Autodesk Inventor part; units mm, degrees
ref_plane "YZ Plane" through (0, 0, 0) normal (1, 0, 0) x (0, 1, 0)
ref_plane "XZ Plane" through (0, 0, 0) normal (0, 1, 0) x (-1, 0, 0)
ref_plane "XY Plane" through (0, 0, 0) normal (0, 0, 1) x (1, 0, 0)
sketch "Sketch1" plane through (0, 0, 0) normal (0, 0, 1) x (1, 0, 0)
  line L0 (0, 0) -> (35, 0)
  line L1 (35, 0) -> (35, 35)
  line L2 (35, 35) -> (0, 35)
  line L3 (0, 35) -> (0, 0)
  line L4 (17.5, 35) -> (17.5, 0)
  line L5 (0, 17.5) -> (35, 17.5)
  dimension "d0" = 35
  dimension "d1" = 35
extrude "Extrusion1" add sketch "Sketch1" along normal blind 10
sketch "Sketch2" plane through (0, 0, 10) normal (0, 0, 1) x (1, 0, 0)
  point P0 (0, 0)
sketch "Sketch3" plane through (0, 0, 10) normal (0, 0, 1) x (1, 0, 0)
  circle A0 centre (17.4625, 15.875) radius 13.5
  point P0 (0, 0)
  dimension "d4" = 27
extrude "Extrusion2" cut sketch "Sketch3" against normal through all
thread "Thread1"
properties part number "dc motor nut"
Could you check a few things on this model? Use its own coordinates, in mm. Round coordinates to 2 decimals unless told otherwise and drop trailing zeros. Write each loop counter-clockwise with the first axis right and the second up, starting at its lowest first coordinate (ties: lowest second). Pieces come first, ordered by that corner, then holes. Notation, with made-up numbers: (77, 79.5) -> (114, 79.5) arc R16 cw to (114, 109.5) -> close; hole circle Ø11 at (-39.5, 11.5). An arc over 180 degrees is marked (long way). Use a Markdown table: item, result.
1. If we section it at A-A (x = 29): List the corners of the cut face in (y, z) for me.
Answer key:
| item | result |
|---|---|
| outline | (0, 0) -> (8.87, 0) -> (8.87, 10) -> (0, 10) -> close; (22.88, 0) -> (35, 0) -> (35, 10) -> (22.88, 10) -> close |
2. Please list where these lines run through material, in increasing order: probe 1 along Y at (x, z) = (17, 2.5); probe 2 along Y at (x, z) = (24.5, 6.75); probe 3 along X at (y, z) = (8, 4.75).
Answer key:
| item | result |
|---|---|
| probe 1 | y = 0 to 2.38, 29.37 to 35 |
| probe 2 | y = 0 to 4.35, 27.4 to 35 |
| probe 3 | x = 0 to 6.5, 28.43 to 35 |
3. We'd pull the mould along Y, two halves only. Please class faces 1 (the face through (17, 0, 5)), 2 (the face through (3.976, 16.469, 5.07)), 3 (the face through (35, 17, 5)): +Y half, -Y half, draft (parallel to the pull), parting line (faces both ways), or undercut.
Answer key:
| item | result |
|---|---|
| face 1 | -Y half |
| face 2 | undercut |
| face 3 | draft |
4. For pin 1 Ø8 at (x, y) = (10.5, 11) entering from -Z, with a flat end and sliding along its axis, tell me the tip position at first contact or that it passes through.
Answer key:
| item | result |
|---|---|
| pin 1 | passes through |
5. If we section it at C-C (z = 8.5): List the corners of the cut face in (x, y) for me (1 decimal), then the cut area to 3 significant figures.
Answer key:
| item | result |
|---|---|
| outline | (0, 0) -> (35, 0) -> (35, 35) -> (0, 35) -> close; hole circle Ø27 at (17.5, 15.9) |
| area | 652 mm^2 |
6. If we section it at B-B (y = 6): List the corners of the cut face in (x, z) for me, then the cut area to 3 significant figures.
Answer key:
| item | result |
|---|---|
| outline | (0, 0) -> (8.26, 0) -> (8.26, 10) -> (0, 10) -> close; (26.67, 0) -> (35, 0) -> (35, 10) -> (26.67, 10) -> close |
| area | 166 mm^2 |
